Study the drawing (mm; zero at the part's minimum x, y, z) and answer. Round coordinates to 2 decimals unless told otherwise and drop trailing zeros. Write each loop counter-clockwise with the first axis right and the second up, starting at its lowest first coordinate (ties: lowest second). Pieces come first, ordered by that corner, then holes. Notation, with made-up numbers: (-36, -33.5) -> (22, -33.5) arc R22 ccw to (22, -27.5) -> close; hole circle Ø1 at (33, 69). An arc over 180 degrees is marked (long way). One line per question, with ' | ' between items. Start each with the question number.
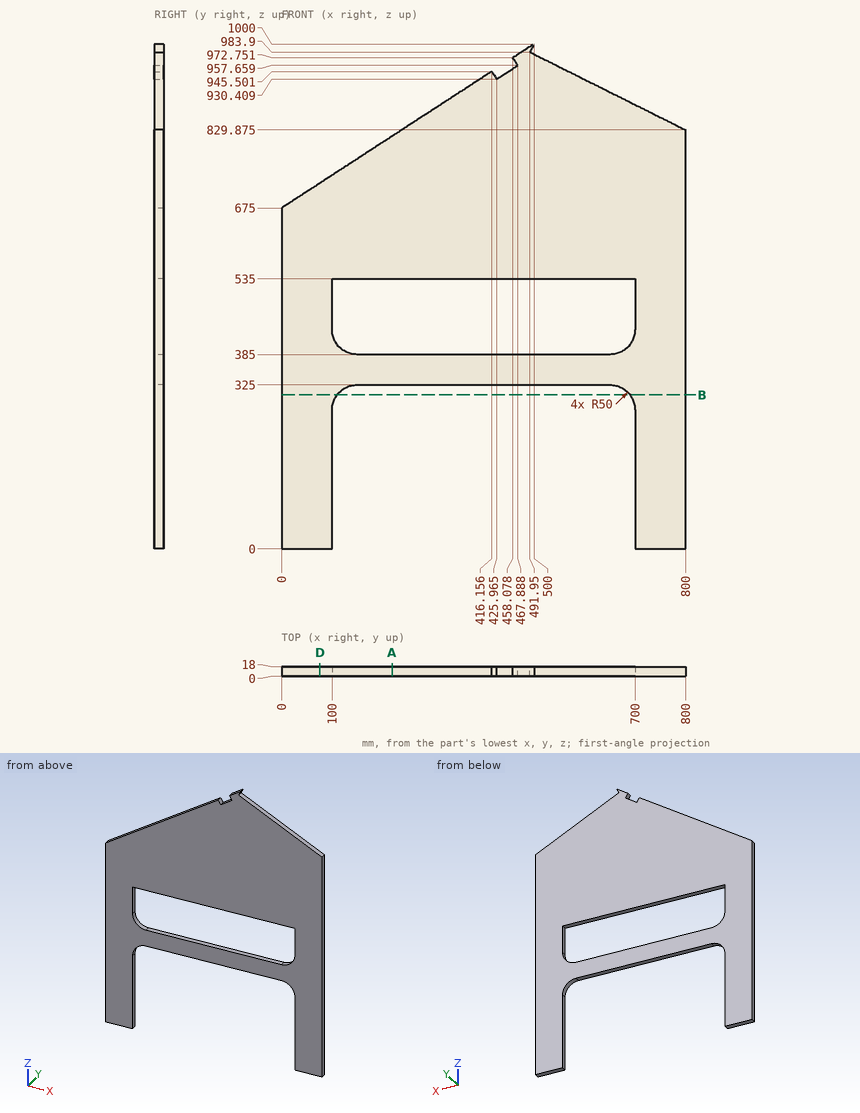
(1) A cutting plane is placed at D-D, the plane x = 76. Determine the outline of the cut face in (y, z), then the cut area to 3 significant figures.
(2) Given pin 1 Ø5.5 at (x, y) = (419, 7.5) entering from -Z; pin 2 Ø4 at (y, z) = (6, 689.5) entering from -X; pin 3 Ø1 at (x, y) = (106.5, 11) entering from +Z, each flat-ended and moving along its own axis, determine where each tip first touches the part or whether it passes through.
(3) A cutting plane is placed at B-B, the plane z = 305. Determine the outline of the cut face in (x, y).
(4) Consider L1, parallel to X at y = 12.5, z = 46.5; L2, parallel to Z at x = 390, y = 1.5. Determine where each line is inside the solid, lowest interval first.
(5) A cutting plane is placed at A-A, the plane x = 219. Determine the outline of the cut face in (y, z).
Returned:
1) outline: (0, 0) -> (18, 0) -> (18, 724.4) -> (0, 724.4) -> close | area: 13,000 mm2
2) pin 1: z = 325 | pin 2: x = 19.23 | pin 3: z = 744.55
3) outline: (0, 0) -> (110, 0) -> (110, 18) -> (0, 18) -> close; (690, 0) -> (800, 0) -> (800, 18) -> (690, 18) -> close
4) L1: 0 to 100, 700 to 800 | L2: 325 to 385, 535 to 928.5
5) outline: (0, 325) -> (18, 325) -> (18, 385) -> (0, 385) -> close; (0, 535) -> (18, 535) -> (18, 817.35) -> (0, 817.35) -> close
